Geometry check sheet. Reference: the model listing, model coordinates, mm. Give positions to 0.01 mm unless a question says otherwise; leave off trailing zeros. Loops run counter-clockwise (first coordinate to the right, second up) from the corner with the lowest first, then second, coordinate; pieces in that order, holes last. Notation, with made-up numbers: (53.25, 22) -> (94.25, 22) arc R28 cw to (94.25, 44) -> close; hole circle Ø6 at (19, 88.5). An arc over 180 degrees is marked (long way). Write item = value, one per line. Start each with the question number.
```python
from build123d import *

# Parameters (mm, degrees)
F0_R     = 8
F1_DEPTH = 3.5
F2_R     = 12.5
F2_R_2   = 7.887929
F3_DEPTH = 1


with BuildPart() as f1:
    # F0 (on Top) → F1 (new body)
    with BuildSketch(Plane.XY):
        with BuildLine():
            ThreePointArc((0, -12.5), (-12.5, 0), (0, 12.5))
            Line((0, 12.5), (-35, 12.5))
            Line((-35, 12.5), (-116.388784, 2.506714))
            Line((-116.388784, 2.506714), (-116.388784, -2.506714))
            Line((-116.388784, -2.506714), (-35, -12.5))
            Line((-35, -12.5), (0, -12.5))
        make_face()
        with BuildLine():
            ThreePointArc((0, -12.5), (8.838835, -8.838835), (12.5, 0))
            ThreePointArc((12.5, 0), (8.838835, 8.838835), (0, 12.5))
            ThreePointArc((0, 12.5), (-12.5, 0), (0, -12.5))
        make_face()
        Circle(F0_R, mode=Mode.SUBTRACT)
    extrude(amount=F1_DEPTH)

    # F2 (on face) → F3 (join)
    with BuildSketch(Plane.XY.offset(3.5)):
        Circle(F2_R)
        Circle(F2_R_2, mode=Mode.SUBTRACT)
    extrude(amount=F3_DEPTH)


solid = f1.part
```
1) Thickness scan on line 1 (Y direction, x = 0, z = 4.1); line 2 (Y direction, x = 0, z = 2.4); line 3 (Z direction, x = -34.5, y = -11.5). Record the ranges inside material, lowest first.
2) Depth check by flat-ended pin: pin 1 Ø5 at (x, y) = (-60.5, -1) entering from +Z; pin 2 Ø2 at (x, y) = (-78, -8.5) entering from -Z. Enter the tip coordinate at first touch or a pass-through.
3) Draft check along X on faces 1 (the flat face through (-39, 0, 0)), 2 (the cylindrical face through (-1.73, -7.81, 1.73)), 3 (the flat face through (-116.389, 0, 2)). Enter one of: released by +X, released by -X, zero draft, split by the parting line, or undercut.
4) Section check C-C (x = -11). Enter the section's corners in (y, z).
5) Section check D-D (y = -10.25). Enter the section's corners in (x, z).
6) Section check B-B (y = 9.5). Enter the section's corners in (x, z).
7) Section check A-A (z = 2.3). Enter the section's corners in (x, y).
Check result:
q1.line_1 = -12.5 to -7.89, 7.89 to 12.5
q1.line_2 = -12.5 to -8, 8 to 12.5
q1.line_3 = 0 to 3.5
q2.pin_1 = 3.5
q2.pin_2 = through
q3.face_1 = zero draft
q3.face_2 = undercut
q3.face_3 = released by -X
q4.outline = (-12.5, 0) -> (12.5, 0) -> (12.5, 3.5) -> (5.94, 3.5) -> (5.94, 4.5) -> (-5.94, 4.5) -> (-5.94, 3.5) -> (-12.5, 3.5) -> close
q5.outline = (-53.32, 0) -> (7.15, 0) -> (7.15, 4.5) -> (-7.15, 4.5) -> (-7.15, 3.5) -> (-53.32, 3.5) -> close
q6.outline = (-59.43, 0) -> (8.12, 0) -> (8.12, 4.5) -> (-8.12, 4.5) -> (-8.12, 3.5) -> (-59.43, 3.5) -> close
q7.outline = (-116.39, -2.51) -> (-35, -12.5) -> (0, -12.5) arc R12.5 ccw to (12.5, 0) arc R12.5 ccw to (0, 12.5) -> (-35, 12.5) -> (-116.39, 2.51) -> close; hole circle Ø16 at (0, 0)
